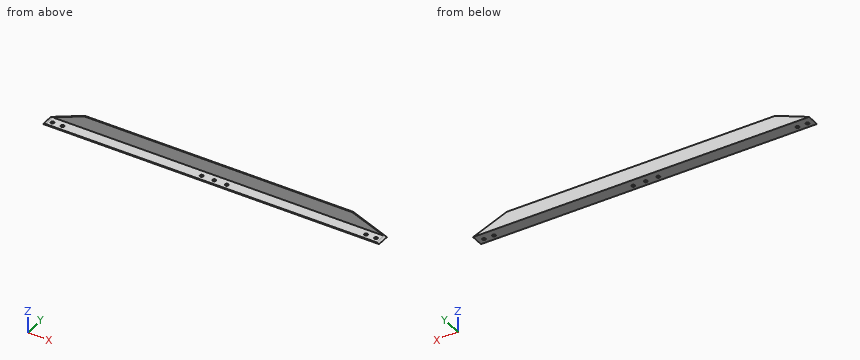
from build123d import *

# Parameters (mm, degrees)
SKETCH_1_W          = 2680
SKETCH_1_H          = 100
SKETCH_1_R          = 13
EXTRUDE_498_DEPTH   = 8
SKETCH_2_W          = 2680
SKETCH_2_H          = 8
EXTRUDE_1_DEPTH     = 100
CUT_EXTRUDE_1_DEPTH = 100


# Read off the part's stored shape, not the designer's step: 切除-拉伸1
with BuildPart() as part:
    # 草图1 → Extrude 498 (new body)
    with BuildSketch(Plane.XY):
        with Locations((0, 50)):
            Rectangle(SKETCH_1_W, SKETCH_1_H)
        with Locations((1290, 40)):
            Circle(SKETCH_1_R, mode=Mode.SUBTRACT)
        with Locations((1210, 40)):
            Circle(SKETCH_1_R, mode=Mode.SUBTRACT)
        with Locations((0, 40)):
            Circle(SKETCH_1_R, mode=Mode.SUBTRACT)
        with Locations((100, 40)):
            Circle(SKETCH_1_R, mode=Mode.SUBTRACT)
        with Locations(Location((-100, 40, 0), (0, 0, 180))):
            Circle(SKETCH_1_R, mode=Mode.SUBTRACT)
        with Locations(Location((-1290, 40, 0), (0, 0, 180))):
            Circle(SKETCH_1_R, mode=Mode.SUBTRACT)
        with Locations(Location((-1210, 40, 0), (0, 0, 180))):
            Circle(SKETCH_1_R, mode=Mode.SUBTRACT)
    extrude(amount=EXTRUDE_498_DEPTH)

    # 草图2 → 凸台-拉伸1 (add)
    with BuildSketch(Plane.XY.offset(8)):
        with Locations((0, 96)):
            Rectangle(SKETCH_2_W, SKETCH_2_H)
    extrude(amount=EXTRUDE_1_DEPTH)

    # 切除-拉伸1 outline → 切除-拉伸1 (cut)
    with BuildSketch(Plane(origin=(0, 0, 0), x_dir=(1, 0, 0), z_dir=(0, 1, 0))):
        Polygon((1340, -108), (1340, 0), (1070, -108), align=None)
        Polygon((-1340, -108), (-1070, -108), (-1340, 0), align=None)
    extrude(amount=CUT_EXTRUDE_1_DEPTH, mode=Mode.SUBTRACT)


solid = part.part
Check sheet for the modelled part. Datum: model origin and axes. Units: mm. Round coordinates to 2 decimals unless told otherwise and drop trailing zeros. Order: outer loops, then holes, each group sorted by start corner. A loop starts at its lowest first (then second) coordinate and runs counter-clockwise, first axis right, second up.
Q1. Cross-section at B-B, the plane x = 614.5. Enter the section's corners in (y, z), plus the area to 3 significant figures.
Filled sheet:
outline: (0, 0) - (100, 0) - (100, 108) - (92, 108) - (92, 8) - (0, 8) - close
area: 1,600 mm2
Q2. Cross-section at A-A, the plane y = 72. Enter the section's corners in (x, z).
Filled sheet:
outline: (-1340, 0) - (1340, 0) - (1320, 8) - (-1320, 8) - close
Q3. Scan lines: L1, parallel to Y at x = -100, z = 4.5; L2, parallel to Y at x = -302, z = 57; L3, parallel to Z at x = 404, y = 44. Record each from-to range of solid material in increasing order.
Filled sheet:
L1: y = 0 to 27, 53 to 100
L2: y = 92 to 100
L3: z = 0 to 8
Q4. Depth check by flat-ended pin: P1, Ø4, axis at x = -13, z = 73, coming from the -Y side. Enter the tip coordinate at first touch or a pass-through.
Filled sheet:
P1: stops at y = 92
Q5. Cross-section at C-C, the plane z = 69. Enter the section's corners in (x, y).
Filled sheet:
outline: (-1167.5, 92) - (1167.5, 92) - (1167.5, 100) - (-1167.5, 100) - close
